Can you work these out from the model? Positions are in its coordinate system, mm. Round coordinates to 2 decimals unless told otherwise and drop trailing zeros. Write each loop counter-clockwise with the first axis right and the second up, starting at its lowest first coordinate (ties: lowest second). Pieces come first, ordered by that corner, then holes. Notation, with made-up numbers: M 5,6.5 L 30,6.5 A30 cw 30,41.5 Z; hole C 64,-17 d3. An arc over 180 degrees is marked long. Answer as a JSON object with one key per item and string values. Group by question number.
1) Suppose I cut it at B-B, the plane y = 79. Write out the boundary of the cut face in (x, z).
2) Please list where these lines run through material, in increasing order: L1, parallel to X at y = 59, z = 2.4; L2, parallel to Y at x = 30, z = 2.15; L3, parallel to X at y = 99.5, z = 2.45. Write a range as [from, to].
3) If we mould it in two halves opening along X, with no side actions, what happens to faces 1 (the cylindrical face through (-39.169, 87.403, 1.479)), 2 (the flat face through (-1, 94, 0))? For each: +X half, -X half, draft (parallel to the pull), parting line (faces both ways), or undercut.
4) Suppose I cut it at C-C, the plane x = -40. State how many separate pieces and enclosed holes the cut face has, and give its area (3 significant figures).
5) Suppose I cut it at A-A, the plane x = 20. Write out the boundary of the cut face in (y, z), and give its area (3 significant figures).
from build123d import *

# Parameters (mm, degrees)
CYLINDER004_R     = 1.8
CYLINDER004_DEPTH = 200
ARRAY003_X_COUNT  = 9
ARRAY003_X_PITCH  = 10
ARRAY003_Y_COUNT  = 2
ARRAY003_Y_PITCH  = 146
CYLINDER006_R     = 1.8
CYLINDER006_DEPTH = 200
ARRAY005_X_COUNT  = 2
ARRAY005_X_PITCH  = 80
ARRAY005_Y_COUNT  = 10
ARRAY005_Y_PITCH  = 10
BOX002_W          = 96
BOX002_H          = 180
BOX002_DEPTH      = 3


with BuildPart() as psu_bottom_bolt_hole_array:
    # Cylinder004 → Cylinder004 (new body)
    with BuildSketch(Plane(origin=(-40, 20, 0), x_dir=(1, 0, 0), z_dir=(0, 0, 1))):
        Circle(CYLINDER004_R)
    extrude(amount=CYLINDER004_DEPTH)

    # Array003 X: psu bottom bolt hole array ×9


with BuildPart() as psu_bottom_bolt_hole_array_1:
    add(psu_bottom_bolt_hole_array.part)
    with Locations(*[(i * ARRAY003_X_PITCH, 0, 0) for i in range(1, ARRAY003_X_COUNT)]):
        add(psu_bottom_bolt_hole_array.part)

    # Array003 Y: psu bottom bolt hole array ×2


with BuildPart() as psu_bottom_bolt_hole_array_2:
    add(psu_bottom_bolt_hole_array_1.part)
    with Locations(*[(0, i * ARRAY003_Y_PITCH, 0) for i in range(1, ARRAY003_Y_COUNT)]):
        add(psu_bottom_bolt_hole_array_1.part)


with BuildPart() as bottom_hole_fusion:
    # Cylinder006 → Cylinder006 (new body)
    with BuildSketch(Plane(origin=(-40, 9, 0), x_dir=(1, 0, 0), z_dir=(0, 0, 1))):
        Circle(CYLINDER006_R)
    extrude(amount=CYLINDER006_DEPTH)

    # Array005 X: bottom hole fusion ×2


with BuildPart() as bottom_hole_fusion_1:
    add(bottom_hole_fusion.part)
    with Locations(*[(i * ARRAY005_X_PITCH, 0, 0) for i in range(1, ARRAY005_X_COUNT)]):
        add(bottom_hole_fusion.part)

    # Array005 Y: bottom hole fusion ×10


with BuildPart() as bottom_hole_fusion_2:
    add(bottom_hole_fusion_1.part)
    with Locations(*[(0, i * ARRAY005_Y_PITCH, 0) for i in range(1, ARRAY005_Y_COUNT)]):
        add(bottom_hole_fusion_1.part)


with BuildPart() as bottom_hole_fusion_3:
    # Array005 placement: moved
    add(bottom_hole_fusion_2.part.moved(Location((0, 40, 0))))

    # Fusion002: union psu bottom bolt hole array
    add(psu_bottom_bolt_hole_array_2.part)


with BuildPart() as psu_bottom_cut:
    # Box002 → Box002 (new body)
    with BuildSketch(Plane(origin=(-48, 3, 0), x_dir=(1, 0, 0), z_dir=(0, 0, 1))):
        with Locations((48, 90)):
            Rectangle(BOX002_W, BOX002_H)
    extrude(amount=BOX002_DEPTH)

    # Cut004: cut bottom hole fusion
    add(bottom_hole_fusion_3.part, mode=Mode.SUBTRACT)


solid = psu_bottom_cut.part
Results:
{
 "1": {"outline": "M -48,0 L -41.8,0 L -41.8,3 L -48,3 Z; M -38.2,0 L 38.2,0 L 38.2,3 L -38.2,3 Z; M 41.8,0 L 48,0 L 48,3 L 41.8,3 Z"},
 "2": {"L1": "[-48, -41.8], [-38.2, 38.2], [41.8, 48]", "L2": "[3, 18.2], [21.8, 164.2], [167.8, 183]", "L3": "[-48, -41.73], [-38.27, 38.27], [41.73, 48]"},
 "3": {"face 1": "undercut", "face 2": "draft"},
 "4": {"separate pieces": "13", "enclosed holes": "0", "area": "410 mm^2"},
 "5": {"outline": "M 3,0 L 18.2,0 L 18.2,3 L 3,3 Z; M 21.8,0 L 164.2,0 L 164.2,3 L 21.8,3 Z; M 167.8,0 L 183,0 L 183,3 L 167.8,3 Z", "area": "518 mm^2"}
}
